from build123d import *

# Parameters (mm, degrees)
SKETCH_2_W          = 8
SKETCH_2_H          = 12
EXTRUDE_1_DEPTH     = 1.5
EXTRUDE_1_2_DEPTH   = 1.5
SKETCH_3_W          = 2
SKETCH_3_H          = 8
EXTRUDE_2_DEPTH     = 24.5
FILLET_1_R          = 4
FILLET_2_R          = 4
SKETCH_4_R          = 1.5
CUT_EXTRUDE_1_DEPTH = 90.622820755
EXTRUDE_3_DEPTH     = 1.5
SKETCH_8_W          = 22
SKETCH_8_H          = 2
EXTRUDE_4_DEPTH     = 4
SKETCH_9_W          = 20
SKETCH_9_H          = 3
CUT_EXTRUDE_2_DEPTH = 61.675365801
FILLET_4_R          = 2
CUT_EXTRUDE_4_DEPTH = 4
FILLET_5_R          = 1
FILLET_6_R          = 1


with BuildPart() as part:
    # Sketch 2 → Extrude 1 (new body)
    with BuildSketch(Plane(origin=(0, 0, 0), x_dir=(1, 0, 0), z_dir=(0, 1, 0))):
        with Locations((-39, 0)):
            Rectangle(SKETCH_2_W, SKETCH_2_H)
    extrude(amount=EXTRUDE_1_DEPTH)



with BuildPart() as body_2:
    # Sketch 2 → Extrude 1 2 (new body)
    with BuildSketch(Plane(origin=(0, 0, 0), x_dir=(1, 0, 0), z_dir=(0, 1, 0))):
        with Locations((39, 0)):
            Rectangle(SKETCH_2_W, SKETCH_2_H)
    extrude(amount=EXTRUDE_1_2_DEPTH)


with BuildPart() as part_1:
    add(part.part)

    add(body_2.part)  # Extrude 2 merges body 2
    # Sketch 3 → Extrude 2 (add)
    with BuildSketch(Plane(origin=(0, 0, 0), x_dir=(1, 0, 0), z_dir=(0, 1, 0))):
        with Locations((-37, 0)):
            Rectangle(SKETCH_3_W, SKETCH_3_H)
        with Locations((-41, 0)):
            Rectangle(SKETCH_3_W, SKETCH_3_H)
        with Locations((41, 0)):
            Rectangle(SKETCH_3_W, SKETCH_3_H)
        with Locations((37, 0)):
            Rectangle(SKETCH_3_W, SKETCH_3_H)
    extrude(amount=-EXTRUDE_2_DEPTH)

    # Fillet 1
    fillet_1_edges = [part_1.edges().sort_by_distance(p)[0] for p in [
        (-41, -24.5, -4),
        (-37, -24.5, -4),
        (-37, -24.5, 4),
        (-41, -24.5, 4),
    ]]
    fillet(fillet_1_edges, radius=FILLET_1_R - 0.0001)  # a hair under: the kernel refuses the full size

    # Fillet 2
    fillet_2_edges = [part_1.edges().sort_by_distance(p)[0] for p in [
        (37, -24.5, 4),
        (41, -24.5, 4),
        (41, -24.5, -4),
        (37, -24.5, -4),
    ]]
    fillet(fillet_2_edges, radius=FILLET_2_R - 0.0001)  # a hair under: the kernel refuses the full size

    # Sketch 4 → Cut-Extrude 1 (cut, through all)
    with BuildSketch(Plane(origin=(43, 0, 0), x_dir=(0, 0, -1), z_dir=(1, 0, 0))):
        with Locations((0, -20.5)):
            Circle(SKETCH_4_R)
    extrude(amount=-CUT_EXTRUDE_1_DEPTH, mode=Mode.SUBTRACT)

    # Sketch 6 → Extrude 3 (add)
    with BuildSketch(Plane(origin=(0, 0, 0), x_dir=(1, 0, 0), z_dir=(0, 1, 0))):
        with BuildLine():
            Line((48.5, -2), (48.5, -40))
            ThreePointArc((48.5, -40), (47.914213562, -41.414213562), (46.5, -42))
            Line((46.5, -42), (35, -42))
            add(Edge.make_bspline(
                [(-35, -42), (0, 5.776780805), (35, -42)],
                knots=[0, 0, 0, 1, 1, 1], degree=2))
            Line((-35, -42), (-46.5, -42))
            ThreePointArc((-46.5, -42), (-47.914213562, -41.414213562), (-48.5, -40))
            Line((-48.5, -40), (-48.5, -2))
            ThreePointArc((-48.5, -2), (-45.571067812, 5.071067812), (-38.5, 8))
            Line((-38.5, 8), (-35, 8))
            add(Edge.make_bspline(
                [(-35, 8), (0, -8), (35, 8)],
                knots=[0, 0, 0, 1, 1, 1], degree=2))
            Line((35, 8), (38.5, 8))
            ThreePointArc((38.5, 8), (45.571067812, 5.071067812), (48.5, -2))
        make_face()
        with BuildLine():
            Line((-43.5, -18.5), (-43.5, -38.5))
            ThreePointArc((-43.5, -38.5), (-45, -40), (-46.5, -38.5))
            Line((-46.5, -38.5), (-46.5, -18.5))
            ThreePointArc((-46.5, -18.5), (-45, -17), (-43.5, -18.5))
        make_face(mode=Mode.SUBTRACT)
        with BuildLine():
            Line((46.5, -18.5), (46.5, -38.5))
            ThreePointArc((46.5, -38.5), (45, -40), (43.5, -38.5))
            Line((43.5, -38.5), (43.5, -18.5))
            ThreePointArc((43.5, -18.5), (45, -17), (46.5, -18.5))
        make_face(mode=Mode.SUBTRACT)
    extrude(amount=EXTRUDE_3_DEPTH)

    # Sketch 8 → Extrude 4 (add)
    with BuildSketch(Plane(origin=(0, 0, 0), x_dir=(-1, 0, 0), z_dir=(0, -1, 0))):
        with Locations((0, -3)):
            Rectangle(SKETCH_8_W, SKETCH_8_H)
        with Locations((0, -14)):
            Rectangle(SKETCH_8_W, SKETCH_8_H)
    extrude(amount=EXTRUDE_4_DEPTH)

    # Sketch 9 → Cut-Extrude 2 (cut, through all)
    with BuildSketch(Plane.XY.offset(15)):
        with Locations((0, -1.5)):
            Rectangle(SKETCH_9_W, SKETCH_9_H)
    extrude(amount=-CUT_EXTRUDE_2_DEPTH, mode=Mode.SUBTRACT)

    # Fillet 4
    fillet_4_edges = [part_1.edges().sort_by_distance(p)[0] for p in [
        (-35, 0.75, -8),
        (35, 0.75, -8),
        (35, 0.75, 42),
        (-35, 0.75, 42),
    ]]
    fillet(fillet_4_edges, radius=FILLET_4_R)

    # Sketch 13 → Cut-Extrude 4 (cut)
    with BuildSketch(Plane(origin=(0, 1.5, 0), x_dir=(1, 0, 0), z_dir=(0, 1, 0))):
        with BuildLine():
            Line((-41.25, -32.200961894), (-15.269237886, -17.200961894))
            ThreePointArc((-15.269237886, -17.200961894), (-13.220199781, -17.75), (-13.769237886, -19.799038106))
            Line((-13.769237886, -19.799038106), (-39.75, -34.799038106))
            ThreePointArc((-39.75, -34.799038106), (-41.799038106, -34.25), (-41.25, -32.200961894))
        make_face()
        with BuildLine():
            Line((-41.25, -26.889339418), (-15.269237886, -11.889339418))
            ThreePointArc((-15.269237886, -11.889339418), (-13.220199781, -12.438377523), (-13.769237886, -14.487415629))
            Line((-13.769237886, -14.487415629), (-39.75, -29.487415629))
            ThreePointArc((-39.75, -29.487415629), (-41.799038106, -28.938377523), (-41.25, -26.889339418))
        make_face()
        with BuildLine():
            Line((-41.25, -21.577716941), (-15.269237886, -6.577716941))
            ThreePointArc((-15.269237886, -6.577716941), (-13.220199781, -7.126755047), (-13.769237886, -9.175793153))
            Line((-13.769237886, -9.175793153), (-39.75, -24.175793153))
            ThreePointArc((-39.75, -24.175793153), (-41.799038106, -23.626755047), (-41.25, -21.577716941))
        make_face()
        with BuildLine():
            Line((-41.25, -16.266094465), (-15.269237886, -1.266094465))
            ThreePointArc((-15.269237886, -1.266094465), (-13.220199781, -1.81513257), (-13.769237886, -3.864170676))
            Line((-13.769237886, -3.864170676), (-39.75, -18.864170676))
            ThreePointArc((-39.75, -18.864170676), (-41.799038106, -18.31513257), (-41.25, -16.266094465))
        make_face()
        with BuildLine():
            Line((-41.25, -10.492591773), (-23.929491924, -0.492591773))
            ThreePointArc((-23.929491924, -0.492591773), (-21.880453819, -1.041629878), (-22.429491924, -3.090667984))
            Line((-22.429491924, -3.090667984), (-39.75, -13.090667984))
            ThreePointArc((-39.75, -13.090667984), (-41.799038106, -12.541629878), (-41.25, -10.492591773))
        make_face()
        with BuildLine():
            Line((-7, -5.75), (7, -5.75))
            ThreePointArc((7, -5.75), (9.75, -8.5), (7, -11.25))
            Line((7, -11.25), (-7, -11.25))
            ThreePointArc((-7, -11.25), (-9.75, -8.5), (-7, -5.75))
        make_face()
        with BuildLine():
            Line((41.25, -32.200961894), (15.269237886, -17.200961894))
            ThreePointArc((15.269237886, -17.200961894), (13.220199781, -17.75), (13.769237886, -19.799038106))
            Line((13.769237886, -19.799038106), (39.75, -34.799038106))
            ThreePointArc((39.75, -34.799038106), (41.799038106, -34.25), (41.25, -32.200961894))
        make_face()
        with BuildLine():
            Line((41.25, -26.889339418), (15.269237886, -11.889339418))
            ThreePointArc((15.269237886, -11.889339418), (13.220199781, -12.438377523), (13.769237886, -14.487415629))
            Line((13.769237886, -14.487415629), (39.75, -29.487415629))
            ThreePointArc((39.75, -29.487415629), (41.799038106, -28.938377523), (41.25, -26.889339418))
        make_face()
        with BuildLine():
            Line((41.25, -21.577716941), (15.269237886, -6.577716941))
            ThreePointArc((15.269237886, -6.577716941), (13.220199781, -7.126755047), (13.769237886, -9.175793153))
            Line((13.769237886, -9.175793153), (39.75, -24.175793153))
            ThreePointArc((39.75, -24.175793153), (41.799038106, -23.626755047), (41.25, -21.577716941))
        make_face()
        with BuildLine():
            Line((41.25, -16.266094465), (15.269237886, -1.266094465))
            ThreePointArc((15.269237886, -1.266094465), (13.220199781, -1.81513257), (13.769237886, -3.864170676))
            Line((13.769237886, -3.864170676), (39.75, -18.864170676))
            ThreePointArc((39.75, -18.864170676), (41.799038106, -18.31513257), (41.25, -16.266094465))
        make_face()
        with BuildLine():
            Line((41.25, -10.492591773), (23.929491924, -0.492591773))
            ThreePointArc((23.929491924, -0.492591773), (21.880453819, -1.041629878), (22.429491924, -3.090667984))
            Line((22.429491924, -3.090667984), (39.75, -13.090667984))
            ThreePointArc((39.75, -13.090667984), (41.799038106, -12.541629878), (41.25, -10.492591773))
        make_face()
    extrude(amount=-CUT_EXTRUDE_4_DEPTH, mode=Mode.SUBTRACT)

    # Fillet 5
    fillet_5_edges = [part_1.edges().sort_by_distance(p)[0] for p in [
        (36, 0, 0),
        (42, 0, 0),
        (-36, 0, 0),
        (-42, 0, 0),
    ]]
    fillet(fillet_5_edges, radius=FILLET_5_R)

    # Fillet 6
    fillet_6_edges = [part_1.edges().sort_by_distance(p)[0] for p in [
        (11, -4, 3),
        (-11, -4, 3),
        (11, -4, 14),
        (-11, -4, 14),
    ]]
    fillet(fillet_6_edges, radius=FILLET_6_R)


solid = part_1.part
Check sheet for the modelled part. Datum: model origin and axes. Units: mm. A direction names the side the tool comes from. Round coordinates to 2 decimals unless told otherwise and drop trailing zeros. Loops run counter-clockwise (first coordinate to the right, second up) from the corner with the lowest first, then second, coordinate; pieces in that order, holes last. Notation, with made-up numbers: (-18, 29.25) -> (36, 29.25) arc R9 ccw to (36, 43.25) -> close; hole circle Ø5 at (49.25, 21). An arc over 180 degrees is marked (long way). Put each result on its own line as item: value. Start each with the question number.
1. Section check C-C (z = 36). Give the number of separate pieces and of enclosed holes in the cut face, plus the area to 3 significant figures.
2. Draft check along X on faces 4 (the face through (11, -1, 3)), 5 (the face through (37.014, -23.297, -2.859)), 6 (the face through (-47.9, 0.74, 41.43)). Enter one of: +X half, -X half, draft (parallel to the pull), parting line (faces both ways), or undercut.
3. Section check B-B (x = -45). Enter the section's corners in (y, z), plus the area to 3 significant figures.
4. Gauge pin test, flat ends, axial feed: pin 1 (9 mm diameter, centred on y = -14, z = 0, fed in from -X); pin 2 (3.5 mm diameter, centred on x = -36.5, y = -15, fed in from -Z); pin 3 (5 mm diameter, centred on x = 16, z = 18, fed in from -Y). Record the tip position at first contact, or that the pin passes through.
5. Scan lines: probe 1 along Y at (x, z) = (-37, 0); probe 2 along Y at (x, z) = (5.5, 3); probe 3 along Y at (x, z) = (-24, 28). Record each from-to range of solid material in increasing order.
6. Section check A-A (y = -6.25). Enter the section's corners in (x, z), plus the area to 3 significant figures.
7. Access from +Z, -Z, +X, -X, +Y, -Y to the whole of each face (thin tool, end or side, straight path). Record for faces 1 (the face through (26.58, 0.76, 11.26)), 2 (the face through (0, -4, 3)), 3 (the face through (-10, -2, 14)).
Findings:
1. separate pieces: 4
1. enclosed holes: 0
1. area: 45.6 mm^2
2. face 4: undercut
2. face 5: draft
2. face 6: -X half
3. outline: (0, -5.6) -> (1.5, -5.6) -> (1.5, 17) -> (0, 17) -> close; (0, 40) -> (1.5, 40) -> (1.5, 42) -> (0, 42) -> close
3. area: 36.9 mm^2
4. pin 1: stops at x = -42
4. pin 2: stops at z = -4
4. pin 3: stops at y = 0
5. probe 1: y = -24.5 to -22, -19 to 1.5
5. probe 2: y = -4 to -3, 0 to 1.5
5. probe 3: y = 0 to 1.5
6. outline: (-42, -4) -> (-40, -4) -> (-40, 4) -> (-42, 4) -> close; (-38, -4) -> (-36, -4) -> (-36, 4) -> (-38, 4) -> close; (36, -4) -> (38, -4) -> (38, 4) -> (36, 4) -> close; (40, -4) -> (42, -4) -> (42, 4) -> (40, 4) -> close
6. area: 64.0 mm^2
7. face 1: +Y, -Y
7. face 2: +Z, -Z, -Y
7. face 3: +Z, -Z
